Check sheet for the drawn part. Datum: minimum x, y, z corner. Units: mm. Round coordinates to 2 decimals unless told otherwise and drop trailing zeros. Write each loop counter-clockwise with the first axis right and the second up, starting at its lowest first coordinate (ties: lowest second). Pieces come first, ordered by that corner, then holes. Notation, with made-up numbers: M -21.5,83.25 L -4.5,83.25 A22 ccw -4.5,108.25 Z; hole C 71.25,-19 d10. An arc over 180 degrees is marked long. One line per item, written item: value.
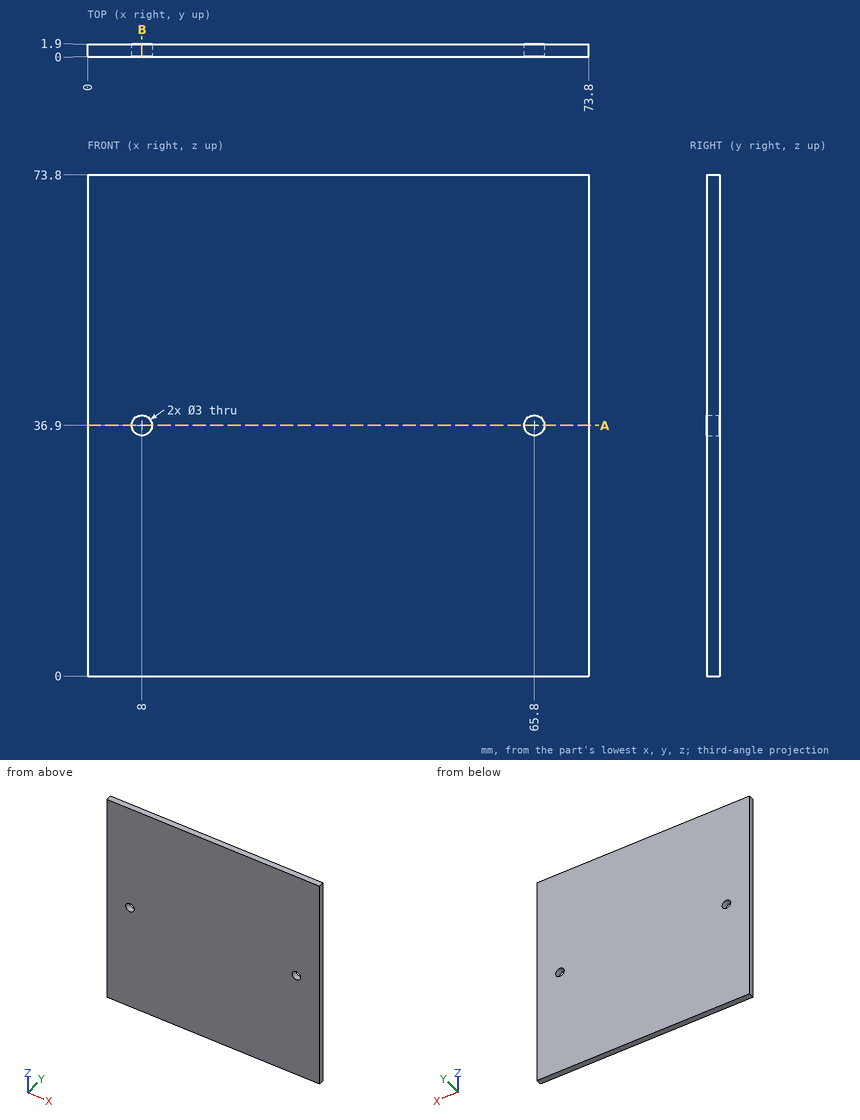
Q1. Depth check by flat-ended pin: P1, Ø4, axis at x = 19.5, z = 50.5, coming from the -Y side. Enter the tip coordinate at first touch or a pass-through.
Completed:
P1: y = 0
Q2. Scan lines: line 1 (X direction, y = 0.65, z = 36.9); line 2 (Z direction, x = 8, y = 0.85); line 3 (Z direction, x = 9, y = 1). Record each from-to range of solid material in increasing order. Write a range as [from, to].
Completed:
line 1: [0, 6.5], [9.5, 64.3], [67.3, 73.8]
line 2: [0, 35.4], [38.4, 73.8]
line 3: [0, 35.78], [38.02, 73.8]
Q3. Sectioned sample at B-B on x = 8. Enter the section's corners in (y, z), and give its area (3 significant figures).
Completed:
outline: M 0,0 L 1.9,0 L 1.9,35.4 L 0,35.4 Z; M 0,38.4 L 1.9,38.4 L 1.9,73.8 L 0,73.8 Z
area: 135 mm^2
Q4. Sectioned sample at A-A on z = 36.9. Enter the section's corners in (x, y).
Completed:
outline: M 0,0 L 6.5,0 L 6.5,1.9 L 0,1.9 Z; M 9.5,0 L 64.3,0 L 64.3,1.9 L 9.5,1.9 Z; M 67.3,0 L 73.8,0 L 73.8,1.9 L 67.3,1.9 Z
